Autodesk Inventor part; units mm, degrees
ref_plane "YZ Plane" through (0, 0, 0) normal (1, 0, 0) x (0, 1, 0)
ref_plane "XZ Plane" through (0, 0, 0) normal (0, 1, 0) x (-1, 0, 0)
ref_plane "XY Plane" through (0, 0, 0) normal (0, 0, 1) x (1, 0, 0)
sketch "Sketch1" plane through (0, 0, 0) normal (0, 0, 1) x (1, 0, 0)
  circle A0 centre (-0.7751, 114.3) radius 2.1844
  circle A1 centre (-0.7751, 139.7) radius 2.1844
  circle A2 centre (202.4249, 139.7) radius 2.1844
  circle A3 centre (202.4249, 114.3) radius 2.1844
  arc A4 (-5.2201, 114.3) -> (-0.7751, 109.855) centre (-0.7751, 114.3) ccw
  circle A5 centre (-0.7751, 139.7) radius 4.445
  arc A6 (206.8699, 139.7) -> (198.7471, 142.1965) centre (202.4249, 139.7) ccw
  arc A7 (202.4249, 109.855) -> (206.8699, 114.3) centre (202.4249, 114.3) ccw
  line L0 (202.4249, 109.855) -> (-0.7751, 109.855)
  line L1 (-5.2201, 114.3) -> (-5.2201, 139.7)
  line L2 (2.9026, 142.1965) -> (10.9801, 130.2968)
  line L3 (13.607, 128.905) -> (188.0427, 128.905)
  line L4 (190.6696, 130.2968) -> (198.7471, 142.1965)
  line L5 (206.8699, 140.9911) -> (206.8699, 114.3)
  arc A8 (188.0427, 128.905) -> (190.6696, 130.2968) centre (188.0427, 132.08) ccw
  arc A9 (10.9801, 130.2968) -> (13.607, 128.905) centre (13.607, 132.08) ccw
  point P0 (0, 0)
  point P1 (11.9249, 128.905)
  point P2 (189.7249, 128.905)
  dimension "d0" = 8.89
  dimension "d2" = 19.05
  dimension "d3" = 177.8
  dimension "d4" = 3.175
extrude "Extrusion1" add sketch "Sketch1" along normal blind 6.35
properties part number "brace" material "Acetal Resin, Black"
Model file for the job. Use its own axes, mm. A direction names the side the tool comes from. Give positions to 0.01 mm unless a question says otherwise; leave off trailing zeros. Write each loop counter-clockwise with the first axis right and the second up, starting at its lowest first coordinate (ties: lowest second). Pieces come first, ordered by that corner, then holes. Notation, with made-up numbers: M 63.25,4 L 114.25,4 A20 ccw 114.25,31 Z; hole C -11.5,-30.5 d11. An arc over 180 degrees is marked long. One line per item, written item: value. Start each with the question number.
Q1. Saw through at A-A, the plane z = 3. Write the cut outline in (x, y) (1 decimal), plus the area to 3 significant figures.
Q2. Two-plate mould, pull along Y, no slides. Class faces 3 (the cylindrical face through (0.23, 141.64, 3.13)), 4 (the cylindrical face through (-2.156, 143.925, 3.131)), 5 (the flat face through (206.87, 127, 3)): +Y half, -Y half, draft (parallel to the pull), parting line (faces both ways), or undercut.
Q3. Saw through at B-B, the plane y = 135.5. Write the cut outline in (x, z), plus the area to 3 significant figures.
Q4. Probe probe 1 along X at (y, z) = (114.5, 6); probe 2 along X at (y, z) = (115.5, 1); probe 3 along X at (y, z) = (139.7, 3). List the from-to ranges inside material, lowest first. Write a range as [from, to].
Q5. 3-axis set-ups, long thin cutter, end or side, ignore diameter. For faces 1 (the flat face through (6.885, 136.33, 3.131)), 2 (the cylindrical face through (-1.249, 116.432, 3.131)): which of +Z, -Z, +X, -X, +Y, -Y reach the whole face in a straight line?
Q6. Saw through at C-C, the plane x = 125.5. Write the cut outline in (y, z) (3 decimals).
Q7. Drop flat-ended pins along their axis: pin 1 Ø1.5 at (x, z) = (142, 2) entering from +Y (3 decimals); pin 2 Ø2.5 at (x, y) = (202.42, 139.7) entering from -Z. Give the stop position or say it passes through.
Output values:
1. outline: M -5.2,114.3 A4.4 ccw -0.8,109.9 L 202.4,109.9 A4.4 ccw 206.9,114.3 L 206.9,139.7 A4.4 ccw 198.7,142.2 L 190.7,130.3 A3.2 cw 188,128.9 L 13.6,128.9 A3.2 cw 11,130.3 L 2.9,142.2 A4.4 ccw -5.2,139.7 Z; hole C -0.8,114.3 d4.4; hole C -0.8,139.7 d4.4; hole C 202.4,114.3 d4.4; hole C 202.4,139.7 d4.4
1. area: 4,330 mm²
2. face 3: undercut
2. face 4: +Y half
2. face 5: draft
3. outline: M -5.22,0 L 7.45,0 L 7.45,6.35 L -5.22,6.35 Z; M 194.2,0 L 206.87,0 L 206.87,6.35 L 194.2,6.35 Z
3. area: 161 mm²
4. probe 1: x = [-5.22, -2.95], [1.4, 200.25], [204.6, 206.87]
4. probe 2: x = [-5.22, -2.6], [1.05, 200.6], [204.25, 206.87]
4. probe 3: x = [-5.22, -2.96], [1.41, 4.6], [197.05, 200.24], [204.61, 206.87]
5. face 1: +Z, -Z, +Y
5. face 2: +Z, -Z
6. outline: M 109.855,0 L 128.905,0 L 128.905,6.35 L 109.855,6.35 Z
7. pin 1: stops at y = 128.905
7. pin 2: passes through
